CAD build for the part. Positions are in the model's coordinates, mm. A direction names the side the tool comes from. Round coordinates to 2 decimals unless told otherwise and drop trailing zeros. Order: outer loops, then holes, each group sorted by start corner. A loop starts at its lowest first (then second) coordinate and runs counter-clockwise, first axis right, second up. Notation, with made-up numbers: M 42,39 L 47,39 A19 cw 47,43 Z; hole C 60.5,48 d7. An arc over 180 degrees is marked long. Answer as a JSON object with one key per item and string values. Group by question number.
```python
from build123d import *

# Parameters (mm, degrees)
BACKSKETCH_W        = 38.1
BACKSKETCH_H        = 50.8
BACKSKETCH_R        = 1.4732
BACKSKETCH_R_2      = 4.572
BACKSKETCH_R_3      = 1.397
BOSS_EXTRUDE1_DEPTH = 3.0734


with BuildPart() as part:
    # backSketch → Boss-Extrude1 (new body)
    # profile 1 of 3: a face of its own
    with BuildSketch(Plane.XY):
        Polygon((38.1, 50.8), (38.1, 25.4), (41.1734, 25.4), (41.1734, 53.8734), (19.196716748, 53.8734), (19.196716748, 50.8), align=None)
    # profile 2 of 3: a face of its own
    with BuildSketch(Plane.XY):
        Polygon((19.05, 0), (0, 0), (0, 25.4), (-3.0734, 25.4), (-3.0734, -3.0734), (19.05, -3.0734), align=None)
    # profile 3 of 3: a face of its own
    with BuildSketch(Plane.XY):
        with Locations((19.05, 25.4)):
            Rectangle(BACKSKETCH_W, BACKSKETCH_H)
        with Locations((19.196716748, 36.578509469)):
            Circle(BACKSKETCH_R, mode=Mode.SUBTRACT)
        with Locations((13.465150567, 18.677705992)):
            Circle(BACKSKETCH_R_2, mode=Mode.SUBTRACT)
        with Locations((32.475268488, 21.466248377)):
            Circle(BACKSKETCH_R_3, mode=Mode.SUBTRACT)
        with Locations((2.925293214, 2.613087759)):
            Circle(BACKSKETCH_R_3, mode=Mode.SUBTRACT)
    extrude(amount=BOSS_EXTRUDE1_DEPTH)


solid = part.part
```
Item 1: Cut at D-D, the plane x = 6.5. Give the cut face in (y, z).
Item 2: Two-plate mould, pull along X, no slides. Class faces 1 (the face through (19, 26, 3.073)), 2 (the face through (38.1, 13, 2)), 3 (the face through (18.03, 35.68, 1.52)): +X half, -X half, draft (parallel to the pull), parting line (faces both ways), or undercut.
Item 3: Drill centre lines: line 1 (X direction, y = 22.5, z = 2.1); line 2 (Y direction, x = 19, z = 2.45); line 3 (Y direction, x = 3, z = 0.65). Where is each one in solid material? Low to high. Write a range as [from, to].
Item 4: Cut at A-A, the plane x = 16. Give the cut face in (y, z), and give its area (3 significant figures).
Item 5: 3-axis set-ups, long thin cutter, end or side, ignore diameter. For faces 4 (the face through (19.197, 52, 2)), 5 (the face through (3.57, 1.374, 1.515)), 6 (the face through (28, 0, 2)): which of +Z, -Z, +X, -X, +Y, -Y reach the whole face in a straight line?
Item 6: Flat gauge pins, fed straight in: pin 1 Ø1.5 at (y, z) = (7.5, 2) entering from +X; pin 2 Ø2.5 at (x, y) = (19.2, 36.58) entering from -Z; pin 3 Ø1.5 at (y, z) = (39.5, 1) entering from -X; pin 4 Ø0.9 at (y, z) = (52.5, 1) entering from -X. Where does each tip first touch, or does it go through?
Item 7: Cut at C-C, the plane y = 13. Give the cut face in (x, z), and give its area (3 significant figures).
Item 8: Cut at B-B, the plane z = 2.55. Give the cut face in (x, y).
Response values:
{
 "1": {"outline": "M -3.07,0 L 50.8,0 L 50.8,3.07 L -3.07,3.07 Z"},
 "2": {"face 1": "draft", "face 2": "+X half", "face 3": "undercut"},
 "3": {"line 1": "[-3.07, 10.96], [15.97, 31.54], [33.41, 38.1]", "line 2": "[-3.07, 35.12], [38.04, 50.8]", "line 3": "[-3.07, 1.22], [4.01, 50.8]"},
 "4": {"outline": "M -3.07,0 L 14.87,0 L 14.87,3.07 L -3.07,3.07 Z; M 22.48,0 L 50.8,0 L 50.8,3.07 L 22.48,3.07 Z", "area": "142 mm^2"},
 "5": {"face 4": "+Z, -Z, -X, +Y", "face 5": "+Z, -Z", "face 6": "+Z, -Z, +X, -Y"},
 "6": {"pin 1": "x = 38.1", "pin 2": "through", "pin 3": "x = 0", "pin 4": "x = 19.2"},
 "7": {"outline": "M -3.07,0 L 38.1,0 L 38.1,3.07 L -3.07,3.07 Z", "area": "127 mm^2"},
 "8": {"outline": "M -3.07,-3.07 L 19.05,-3.07 L 19.05,0 L 38.1,0 L 38.1,25.4 L 41.17,25.4 L 41.17,53.87 L 19.2,53.87 L 19.2,50.8 L 0,50.8 L 0,25.4 L -3.07,25.4 Z; hole C 2.93,2.61 d2.79; hole C 13.47,18.68 d9.14; hole C 19.2,36.58 d2.95; hole C 32.48,21.47 d2.79"}
}
